Check sheet for the drawn part. Datum: minimum x, y, z corner. Units: mm. A direction names the side the tool comes from. Coordinates: 2 decimals unless noted, no trailing zeros. Order: outer loops, then holes, each group sorted by start corner. A loop starts at its lowest first (then second) coordinate and runs counter-clockwise, first axis right, second up.
Q1. Draft check along Y on the marked faces 6, 7, 8 and 9. Enter one of: pulls with the +Y half, pulls with the -Y half, needs draft (parallel to the pull), parting line crosses it, or undercut.
Q2. Cross-section at A-A, the plane z = 32.5. Record the boundary of the cut face in (x, y), and give its area (3 significant figures).
Q3. Set-up check for the marked faces 1, 2, 3, 4 and 5: record each of +Z, -Z, +X, -X, +Y, -Y from which the full face is reachable in a straight line by a thin tool's end or side.
Q4. Cross-section at C-C, the plane y = 45. Record the boundary of the cut face in (x, z).
Q5. Depth check by flat-ended pin: P1, Ø12, axis at y = 35, z = 21, coming from the +X side; P2, Ø19, axis at x = 41.5, z = 53.5, coming from the +Y side; P3, Ø10, axis at x = 11, y = 44, coming from the -Z side; P4, Ø8.5, axis at x = 5, z = 27.5, coming from the +Y side. Enter the tip coordinate at first touch or a pass-through.
Q6. Thickness scan on line 1 (Y direction, x = 32.5, z = 32.5); line 2 (Z direction, x = 64.5, y = 12); line 3 (X direction, y = 40, z = 51). Record the ranges inside material, lowest first.
Q7. Cross-section at D-D, the plane z = 11.5. Record the boundary of the cut face in (x, y).
Q8. Cross-section at B-B, the plane x = 31. Record the boundary of the cut face in (y, z).
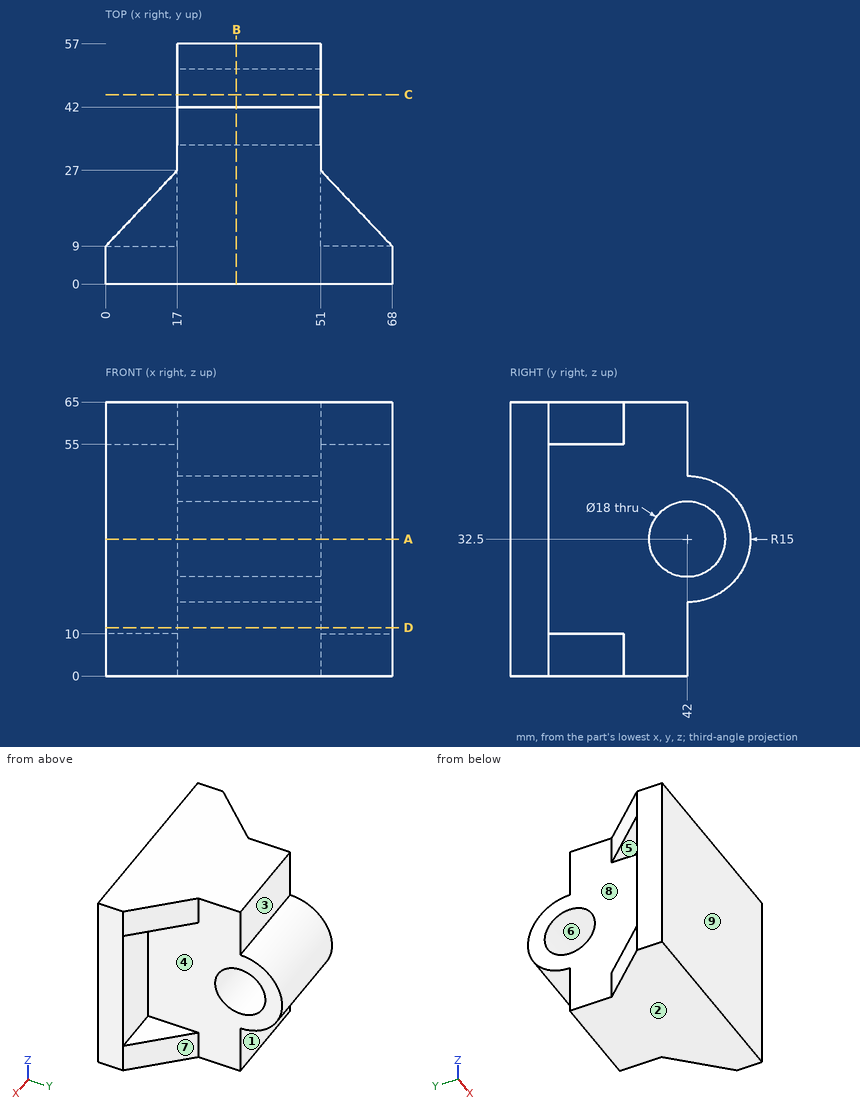
Check values:
1. face 6: undercut
1. face 7: pulls with the +Y half
1. face 8: needs draft
1. face 9: pulls with the -Y half
2. outline: (0, 0) - (68, 0) - (68, 9) - (51, 9) - (51, 33) - (17, 33) - (17, 9) - (0, 9) - close; (17, 51) - (51, 51) - (51, 57) - (17, 57) - close
2. area: 1,630 mm2
3. face 1: -Z, +X, -X, +Y
3. face 2: -Z, +X, -X, +Y, -Y
3. face 3: +Z, +X, -X, +Y
3. face 4: +X, +Y
3. face 5: -X, +Y
4. outline: (17, 17.8) - (51, 17.8) - (51, 24.01) - (17, 24.01) - close; (17, 40.99) - (51, 40.99) - (51, 47.2) - (17, 47.2) - close
5. P1: stops at x = 51
5. P2: stops at y = 51.63
5. P3: passes through
5. P4: stops at y = 9
6. line 1: y = 0 to 33, 51 to 57
6. line 2: z = 0 to 10, 55 to 65
6. line 3: x = 17 to 51
7. outline: (0, 0) - (68, 0) - (68, 9) - (51, 9) - (51, 42) - (17, 42) - (17, 9) - (0, 9) - close
8. outline: (0, 0) - (42, 0) - (42, 17.5) arc R15 ccw to (42, 47.5) - (42, 65) - (0, 65) - close; hole circle Ø18 at (42, 32.5)
